Part model, mm, in its own coordinate system. A direction names the side the tool comes from. Coordinates: 2 decimals unless noted, no trailing zeros. Loops run counter-clockwise (first coordinate to the right, second up) from the corner with the lowest first, then second, coordinate; pieces in that order, holes last. Notation, with made-up numbers: (58, 43.25) -> (101, 43.25) arc R26 cw to (101, 75.25) -> close; hole circle Ø6 at (83.25, 86). An arc over 180 degrees is marked (long way). One line per question, with ' | ' between items. Start each with the question number.
1) 3-axis set-ups, long thin cutter, end or side, ignore diameter. For faces 4 (the face through (-22, -52, 33)), 5 (the face through (-22, 2.5, 17)): which of +Z, -Z, +X, -X, +Y, -Y reach the whole face in a straight line?
2) Cut at B-B (x = -36). List the corners of the cut face in (y, z), plus the area to 3 significant figures.
3) Cut at C-C (y = -55.5). List the corners of the cut face in (x, z), plus the area to 3 significant figures.
4) Cut at A-A (y = -43.5). List the corners of the cut face in (x, z).
5) Cut at D-D (x = -22.5). List the corners of the cut face in (y, z).
6) Two-plate mould, pull along Y, no slides. Class faces 1 (the face through (-22, -23, 33)), 2 (the face through (-22, -49.5, 45)), 3 (the face through (-36.879, -36.542, 32.24)): released by +Y, released by -Y, zero draft, split by the parting line, or undercut.
7) Drop flat-ended pins along their axis: pin 1 (3.5 mm diameter, centred on x = -36, y = -37.5, fed in from -Z); pin 2 (5.5 mm diameter, centred on x = -12, y = -31.5, fed in from +Z); pin 3 (5 mm diameter, centred on x = -18, z = 51, fed in from +Y). Give the stop position or say it passes through.
8) Probe L1, parallel to X at y = -50, z = 39; L2, parallel to X at y = 1, z = 28; L3, parallel to Z at x = -18, y = -50. List the from-to ranges inside material, lowest first. Write a range as from..to.
Autodesk Inventor part; units mm, degrees
ref_plane "YZ Plane" through (0, 0, 0) normal (1, 0, 0) x (0, 1, 0)
ref_plane "XZ Plane" through (0, 0, 0) normal (0, 1, 0) x (-1, 0, 0)
ref_plane "XY Plane" through (0, 0, 0) normal (0, 0, 1) x (1, 0, 0)
sketch "Sketch1" plane through (0, 0, 0) normal (0, 1, 0) x (-1, 0, 0)
  line L0 (0, 0) -> (45, 0)
  line L1 (45, 0) -> (45, 31.5)
  line L2 (45, 31.5) -> (0, 31.5)
  line L3 (0, 31.5) -> (0, 0)
  dimension "d0" = 45
  dimension "d1" = 31.5
extrude "Extrusion1" add sketch "Sketch1" along normal blind 2.5
sketch "Sketch2" plane through (0, 0, 0) normal (0, -1, 0) x (1, 0, 0)
  line L0 (-45, 0) -> (-45, 31.5)
  line L1 (-45, 31.5) -> (0, 31.5)
  line L2 (0, 31.5) -> (0, 33)
  line L3 (0, 33) -> (-45, 33)
  line L4 (-45, 33) -> (-45, 31.5)
  point P0 (0, 0)
  dimension "d4" = 45
  dimension "d5" = 1.5
extrude "Extrusion2" add sketch "Sketch2" along normal blind 60 and the other way blind 2.5
sketch "Sketch4" plane through (0, 0, 0) normal (0, -1, 0) x (1, 0, 0)
  circle A0 centre (-3.5, 28) radius 2.3
  line L0 (-45, 31.5) -> (0, 31.5)
  line L1 (0, 31.5) -> (0, 0)
  line L2 (0, 0) -> (-45, 0)
  circle A1 centre (-41.5, 28) radius 2.3
  line L3 (-45, 0) -> (-45, 31.5)
  circle A2 centre (-41.5, 3.5) radius 2.3
  dimension "d10" = 4.6
  dimension "d11" = 3.5
  dimension "d12" = 3.5
  dimension "d16" = 4.6
  dimension "d17" = 3.5
  dimension "d18" = 3.5
  dimension "d19" = 4.6
  dimension "d20" = 3.5
  dimension "d21" = 3.5
hole "Hole1" at (-3.5, 0, 28) at (-41.5, 0, 28) at (-41.5, 0, 3.5) direction (0, 1, 0) diameter 4.6 end through all
sketch "Sketch5" plane through (-45, -60, 33) normal (0, 0, 1) x (1, 0, 0)
  circle A0 centre (4.5, 4.5) radius 2.15
  line L0 (45, 0) -> (0, 0)
  line L1 (0, 62.5) -> (0, 0)
  circle A1 centre (40.5, 4.5) radius 2.15
  line L2 (45, 62.5) -> (45, 0)
  circle A2 centre (22.5, 4.5) radius 2.15
  point P0 (45, 60)
  dimension "d29" = 4.3
  dimension "d30" = 4.5
  dimension "d31" = 4.5
  dimension "d32" = 4.3
  dimension "d33" = 4.5
  dimension "d34" = 4.5
  dimension "d35" = 4.3
hole "Hole2" at (-40.5, -55.5, 33) at (-4.5, -55.5, 33) at (-22.5, -55.5, 33) direction (0, 0, -1) diameter 4.6 end through all
sketch "Sketch6" plane through (-45, -60, 33) normal (0, 0, 1) x (1, 0, 0)
  circle A0 centre (4.5, 4.5) radius 2.3
  line L0 (4.5, 4.5) -> (4.5, 9)
  line L1 (0, 0) -> (0, 60)
  line L2 (0, 9) -> (45, 9)
  line L3 (45, 9) -> (45, 10.5)
  line L4 (45, 60) -> (45, 0)
  line L5 (45, 10.5) -> (0, 10.5)
  line L6 (0, 10.5) -> (0, 9)
  dimension "d43" = 4.5
  dimension "d44" = 1.5
extrude "Extrusion3" add sketch "Sketch6" along normal blind 24 contours L2 L1 L5 L3
sketch "Sketch7" plane through (-45, 2.5, 33) normal (0, 0, 1) x (1, 0, 0)
  circle A0 centre (9, -40) radius 1.3
  line L0 (0, 0) -> (0, -52)
  line L1 (45, -52) -> (0, -52)
  circle A1 centre (33, -40) radius 2.15
  circle A2 centre (33, -34) radius 2.15
  circle A3 centre (33, -46) radius 2.15
  point P0 (45, -2.5)
  dimension "d47" = 2.6
  dimension "d48" = 9
  dimension "d49" = 12
  dimension "d50" = 4.3
  dimension "d51" = 24
  dimension "d52" = 4.3
  dimension "d53" = 6
  dimension "d54" = 4.3
  dimension "d55" = 6
hole "Hole3" at (-12, -31.5, 33) at (-12, -37.5, 33) at (-12, -43.5, 33) direction (0, 0, -1) diameter 4.3 end through all
sketch "Sketch8" plane through (-45, 2.5, 33) normal (0, 0, 1) x (1, 0, 0)
  circle A0 centre (33, -40) radius 2.15
  line L0 (0, 0) -> (0, -52)
  circle A1 centre (9, -40) radius 1.3
  point P0 (45, -2.5)
  dimension "d89" = 2.6
  dimension "d91" = 9
hole "Hole4" at (-12, -37.5, 33) at (-36, -37.5, 33) direction (0, 0, -1) diameter 2.6 end through all
sketch "Sketch9" plane through (-45, -49.5, 33) normal (0, 1, 0) x (1, 0, 0)
  circle A0 centre (9, -6) radius 2.15
  line L0 (0, 0) -> (45, 0)
  line L1 (0, 0) -> (0, -24)
  circle A1 centre (9, -18) radius 2.15
  circle A2 centre (27, -18) radius 2.15
  circle A3 centre (27, -6) radius 2.15
  point P0 (45, 33)
  dimension "d73" = 4.3
  dimension "d74" = 6
  dimension "d75" = 9
  dimension "d76" = 4.3
  dimension "d77" = 12
  dimension "d78" = 4.3
  dimension "d79" = 18
  dimension "d80" = 4.3
  dimension "d104" = 18
  dimension "d105" = 9
hole "Hole5" at (-36, -49.5, 39) at (-36, -49.5, 51) at (-18, -49.5, 51) at (-18, -49.5, 39) direction (0, -1, 0) diameter 4.3 end through all
sketch "Sketch10" plane through (0, 2.5, 0) normal (0, 1, 0) x (1, 0, 0)
  circle A0 centre (-7.5, -6) radius 1.5
  line L0 (0, 0) -> (-45, 0)
  line L1 (0, -33) -> (0, 0)
  circle A1 centre (-25.5, -6) radius 1.5
  dimension "d92" = 3
  dimension "d93" = 6
  dimension "d94" = 7.5
  dimension "d95" = 3
  dimension "d96" = 18
hole "Hole6" at (-25.5, 2.5, 6) at (-7.5, 2.5, 6) direction (0, -1, 0) diameter 3 end through all
properties part number "TrolleyLeftPlate1"
Reported:
1) face 4: +Z, +X, -X, -Y | face 5: +Z, -Z, +X, -X, +Y
2) outline: (-60, 31.5) -> (-38.8, 31.5) -> (-38.8, 33) -> (-49.5, 33) -> (-49.5, 36.85) -> (-51, 36.85) -> (-51, 33) -> (-60, 33) -> close; (-51, 41.15) -> (-49.5, 41.15) -> (-49.5, 48.85) -> (-51, 48.85) -> close; (-51, 53.15) -> (-49.5, 53.15) -> (-49.5, 57) -> (-51, 57) -> close; (-36.2, 31.5) -> (0, 31.5) -> (0, 0) -> (2.5, 0) -> (2.5, 33) -> (-36.2, 33) -> close | area: 192 mm²
3) outline: (-45, 31.5) -> (-42.8, 31.5) -> (-42.8, 33) -> (-45, 33) -> close; (-38.2, 31.5) -> (-24.8, 31.5) -> (-24.8, 33) -> (-38.2, 33) -> close; (-20.2, 31.5) -> (-6.8, 31.5) -> (-6.8, 33) -> (-20.2, 33) -> close; (-2.2, 31.5) -> (0, 31.5) -> (0, 33) -> (-2.2, 33) -> close | area: 46.8 mm²
4) outline: (-45, 31.5) -> (-14.15, 31.5) -> (-14.15, 33) -> (-45, 33) -> close; (-9.85, 31.5) -> (0, 31.5) -> (0, 33) -> (-9.85, 33) -> close
5) outline: (-60, 31.5) -> (-57.8, 31.5) -> (-57.8, 33) -> (-60, 33) -> close; (-53.2, 31.5) -> (0, 31.5) -> (0, 0) -> (2.5, 0) -> (2.5, 33) -> (-49.5, 33) -> (-49.5, 57) -> (-51, 57) -> (-51, 33) -> (-53.2, 33) -> close
6) face 1: zero draft | face 2: released by +Y | face 3: undercut
7) pin 1: stops at z = 31.5 | pin 2: stops at z = 33 | pin 3: stops at y = -49.5
8) L1: x = -45..-38.15, -33.85..-20.15, -15.85..0 | L2: x = -45..-43.8, -39.2..-5.8, -1.2..0 | L3: z = 31.5..36.85, 41.15..48.85, 53.15..57
